from build123d import *

# Parameters (mm, degrees)
F0_W     = 150
F0_H     = 140
F1_DEPTH = 2
F2_R     = 2.5
F3_DEPTH = 5
F4_R     = 50
F4_R_2   = 49.75
F5_DEPTH = 1


with BuildPart() as f1:
    # F0 (on Top) → F1 (new body)
    with BuildSketch(Plane.XY):
        Rectangle(F0_W, F0_H)
    extrude(amount=F1_DEPTH)

    # F2 (on face) → F3 (cut)
    with BuildSketch(Plane.XY.offset(2)):
        Polygon((-75, 70), (-75, 41.5), (-46.5, 70), align=None)
        with Locations((-64, 57.6)):
            Circle(F2_R, mode=Mode.SUBTRACT)
        Polygon((-46.5, -70), (-75, -41.5), (-75, -70), align=None)
        with Locations((-64, -57.6)):
            Circle(F2_R, mode=Mode.SUBTRACT)
        with BuildLine():
            Line((-67.1845650673, -6.35), (-67.1845650673, 6.35))
            ThreePointArc((-67.1845650673, 6.35), (-67.9167981143, 8.117766953), (-69.6845650673, 8.85))
            Line((-69.6845650673, 8.85), (-75, 8.85))
            Line((-75, 8.85), (-75, -8.85))
            Line((-75, -8.85), (-69.6845650673, -8.85))
            ThreePointArc((-69.6845650673, -8.85), (-67.9167981143, -8.117766953), (-67.1845650673, -6.35))
        make_face()
        with BuildLine():
            Line((-21.499911428, -66.5210440509), (-22.940942165, -70))
            Line((-22.940942165, -70), (-14.8778247705, -70))
            Line((-14.8778247705, -70), (-16.500088572, -66.5210440509))
            ThreePointArc((-16.500088572, -66.5210440509), (-19, -64), (-21.499911428, -66.5210440509))
        make_face()
        with BuildLine():
            Line((-14.8778247705, 70), (-22.940942165, 70))
            Line((-22.940942165, 70), (-21.499911428, 66.5210440509))
            ThreePointArc((-21.499911428, 66.5210440509), (-19, 64), (-16.500088572, 66.5210440509))
            Line((-16.500088572, 66.5210440509), (-14.8778247705, 70))
        make_face()
        with Locations((-64, 57.6)):
            Circle(F2_R)
        with Locations((-64, -57.6)):
            Circle(F2_R)
    extrude(amount=-F3_DEPTH, mode=Mode.SUBTRACT)

    # F4 (on face) → F5 (join)
    with BuildSketch(Plane.XY.offset(2)):
        with Locations((-3.16328, 0)):
            Circle(F4_R)
        with Locations((-3.16328, 0)):
            Circle(F4_R_2, mode=Mode.SUBTRACT)
    extrude(amount=F5_DEPTH)


solid = f1.part
Work out the finished part from the listing and answer in its coordinate system (mm). A direction names the side the tool comes from. Give positions to 0.01 mm unless a question says otherwise; leave off trailing zeros. Order: outer loops, then holes, each group sorted by start corner. A loop starts at its lowest first (then second) coordinate and runs counter-clockwise, first axis right, second up. Notation, with made-up numbers: (10.5, -1.75) -> (39.5, -1.75) arc R22 cw to (39.5, 31.25) -> close; hole circle Ø5 at (11.25, -16). An arc over 180 degrees is marked (long way). One line per item, written item: value.
Item 1: Find section D-D, the plane x = -58.5. Give the vertices of the cut face in (y, z), plus the area to 3 significant figures.
Answer sheet:
outline: (-58, 0) -> (58, 0) -> (58, 2) -> (-58, 2) -> close
area: 232 mm²
Item 2: A tool of negligible diameter and unlimited length cuts with its end or side. For faces 5 (the flat face through (-4, 1, 2)), 6 (the flat face through (-1, 1, 0)), from which of +Z, -Z, +X, -X, +Y, -Y can it reach the whole face along a straight path? Write none if from no direction.
Answer sheet:
face 5: +Z
face 6: -Z, +X, -X, +Y, -Y
Item 3: Find section B-B, the plane x = 26. Give the vertices of the cut face in (y, z), plus the area to 3 significant figures.
Answer sheet:
outline: (-70, 0) -> (70, 0) -> (70, 2) -> (40.61, 2) -> (40.61, 3) -> (40.31, 3) -> (40.31, 2) -> (-40.31, 2) -> (-40.31, 3) -> (-40.61, 3) -> (-40.61, 2) -> (-70, 2) -> close
area: 281 mm²
Item 4: Determine the mould class of faces 1 (the cylindrical face through (44.29, 14.94, 2.49)), 2 (the flat face through (49, 1, 2)), 3 (the flat face through (-60.6, -55.9, 1)), 4 (the cylindrical face through (44.528, 15.019, 2.493)) for opening direction X: released by +X, released by -X, zero draft, split by the parting line, or undercut.
Answer sheet:
face 1: undercut
face 2: zero draft
face 3: released by -X
face 4: split by the parting line
Item 5: Find section C-C, the plane x = 48.5. Give the vertices of the cut face in (y, z), plus the area to 3 significant figures.
Answer sheet:
outline: (-70, 0) -> (70, 0) -> (70, 2) -> (-70, 2) -> close
area: 280 mm²
Item 6: Find section A-A, the plane y = 0. Give the vertices of the cut face in (x, z), plus the area to 3 significant figures.
Answer sheet:
outline: (-67.18, 0) -> (75, 0) -> (75, 2) -> (46.84, 2) -> (46.84, 3) -> (46.59, 3) -> (46.59, 2) -> (-52.91, 2) -> (-52.91, 3) -> (-53.16, 3) -> (-53.16, 2) -> (-67.18, 2) -> close
area: 285 mm²
Item 7: Flat-ended cylindrical pins translate along their axes: P1, Ø1, axis at y = 1, z = 1.5, coming from the -X side; P2, Ø1.5, axis at x = 26.5, y = -1, coming from the +Z side; P3, Ø0.6, axis at x = -71.5, z = 1, coming from the +Y side. Find the tip coordinate at first contact, or state that the pin passes through.
Answer sheet:
P1: x = -67.18
P2: z = 2
P3: y = 45.3
Item 8: Straight lines are drawn through the part: probe 1 along Z at (x, y) = (25, -55.5); probe 2 along X at (y, z) = (-29, 2.35); probe 3 along Y at (x, z) = (9.5, 2.65). For each, find the intervals that lie inside material, in ascending order.
Answer sheet:
probe 1: 0 to 2
probe 2: -43.89 to -43.59, 37.26 to 37.57
probe 3: -48.37 to -48.11, 48.11 to 48.37
